Verification items for this drawing (mm, ordinates from the low corner). A direction names the side the tool comes from. Round coordinates to 2 decimals unless told otherwise and drop trailing zeros. Loops run counter-clockwise (first coordinate to the right, second up) from the corner with the lowest first, then second, coordinate; pieces in that order, holes last. Notation, with made-up numbers: M -9,51.25 L 34,51.25 A21 cw 34,74.25 Z; hole C 8.5,74 d7. An arc over 180 degrees is marked long. Write item = value, one per line.
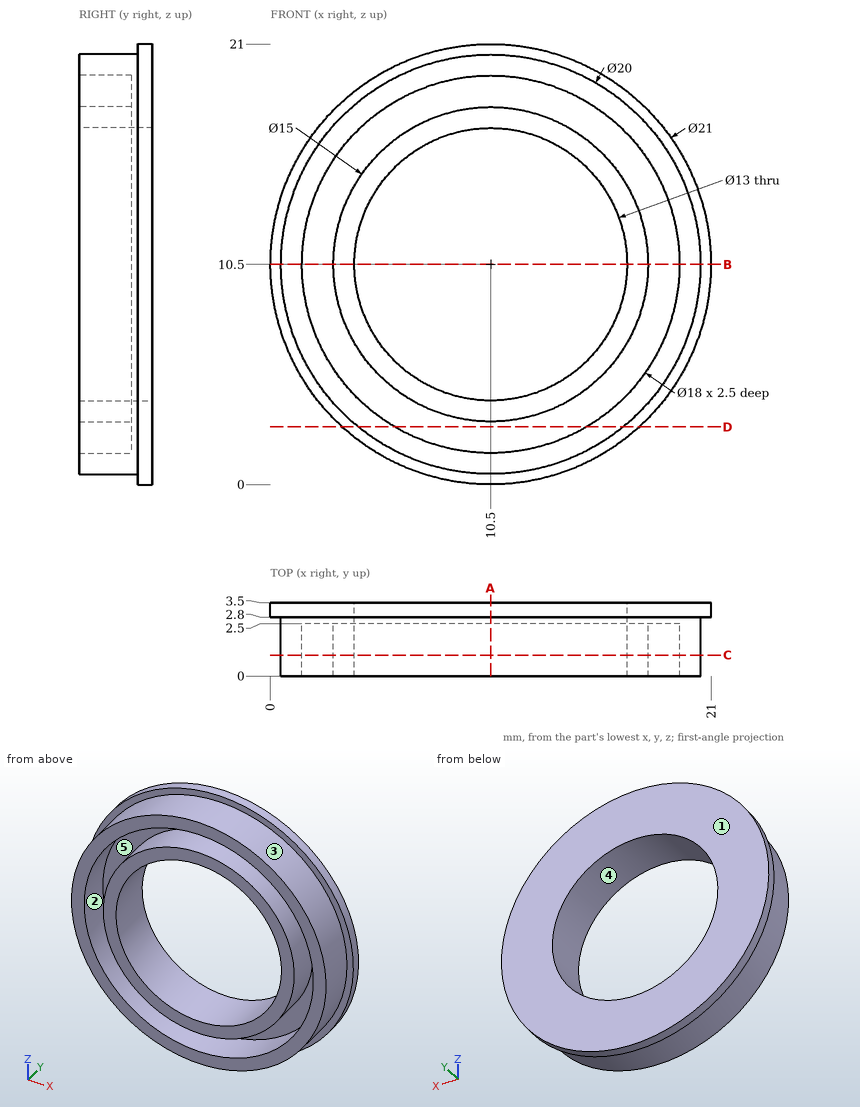
(1) Sectioned sample at D-D on z = 2.75. Record the cut outline in (x, y), then the cut area to 3 significant figures.
Result set:
outline = M 3.42,2.8 L 4.18,2.8 L 4.18,0 L 5.92,0 L 5.92,2.5 L 15.08,2.5 L 15.08,0 L 16.82,0 L 16.82,2.8 L 17.58,2.8 L 17.58,3.5 L 3.42,3.5 Z
area = 22.4 mm2
(2) Release check for a two-part mould opening along X. For the marked faces 1, 2 and 3 record: released by +X, released by -X, zero draft, split by the parting line, or undercut.
Result set:
face_1 = zero draft
face_2 = undercut
face_3 = split by the parting line
(3) Sectioned sample at C-C on y = 1. Record the cut outline in (x, z), then the cut area to 3 significant figures.
Result set:
outline = C 10.5,10.5 d20; C 10.5,10.5 d15; hole C 10.5,10.5 d18; hole C 10.5,10.5 d13
area = 104 mm2
(4) Sectioned sample at A-A on x = 10.5. Record the cut outline in (y, z), then the cut area to 3 significant figures.
Result set:
outline = M 0,0.5 L 2.8,0.5 L 2.8,0 L 3.5,0 L 3.5,4 L 0,4 L 0,3 L 2.5,3 L 2.5,1.5 L 0,1.5 Z; M 0,17 L 3.5,17 L 3.5,21 L 2.8,21 L 2.8,20.5 L 0,20.5 L 0,19.5 L 2.5,19.5 L 2.5,18 L 0,18 Z
area = 17.7 mm2
(5) Material ranges on line 1 along X through (y, z) = (0.5, 10.5); line 2 along Z through (x, y) = (6.25, 2.15); line 3 along Z through (x, y) = (5, 0.7), recorded low to high. Write a range as from..to.
Result set:
line_1 = 0.5..1.5, 3..4, 17..18, 19.5..20.5
line_2 = 1.45..2.57, 4.32..5.58, 15.42..16.68, 18.43..19.55
line_3 = 2.15..3.38, 5.4..7.04, 13.96..15.6, 17.62..18.85
(6) Tool access check on the marked faces 4 and 5. Record the directions out of +Z, -Z, +X, -X, +Y, -Y that give a thin tool (end or side, any length) a straight path to the whole face; none if there is none.
Result set:
face_4 = +Y, -Y
face_5 = -Y
(7) Depth check by flat-ended pin: pin 1 Ø10.5 at (x, z) = (10, 13) entering from -Y. Enter the tip coordinate at first touch or a pass-through.
Result set:
pin_1 = 0
(8) Sectioned sample at B-B on z = 10.5. Record the cut outline in (x, y), then the cut area to 3 significant figures.
Result set:
outline = M 0,2.8 L 0.5,2.8 L 0.5,0 L 1.5,0 L 1.5,2.5 L 3,2.5 L 3,0 L 4,0 L 4,3.5 L 0,3.5 Z; M 17,0 L 18,0 L 18,2.5 L 19.5,2.5 L 19.5,0 L 20.5,0 L 20.5,2.8 L 21,2.8 L 21,3.5 L 17,3.5 Z
area = 17.7 mm2
